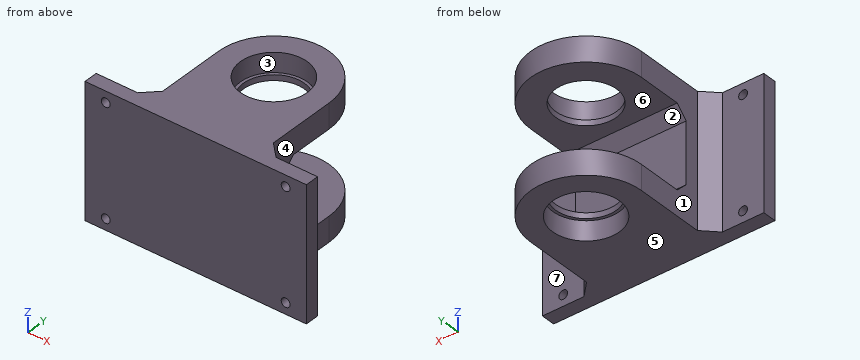
```python
from build123d import *

# Parameters (mm, degrees)
SKETCH_1_R               = 11
EXTRUDE_1_DEPTH          = 24
CUT_EXTRUDE_1_DEPTH      = 47.914816423
CUT_EXTRUDE_1_DEPTH_BACK = 47.914816423
SKETCH_2_W               = 30
SKETCH_2_H               = 69.949963181
SKETCH_4_R               = 12.05
CUT_EXTRUDE_3_DEPTH      = 7
CHAMFER_2_SIZE           = 4
SKETCH_5_W               = 48
SKETCH_5_H               = 5
EXTRUDE_2_DEPTH          = 20
CHAMFER_3_SIZE           = 5
SKETCH_6_R               = 1.6
CUT_EXTRUDE_4_DEPTH      = 73.117958928


with BuildPart() as part:
    # 草图1 → 凸台-拉伸1 (new, symmetric)
    with BuildSketch(Plane.XY):
        with BuildLine():
            Line((-20, -35), (-20, 0))
            ThreePointArc((-20, 0), (0, 20), (20, 0))
            Line((20, 0), (20, -35))
            Line((20, -35), (-20, -35))
        make_face()
        Circle(SKETCH_1_R, mode=Mode.SUBTRACT)
    extrude(amount=EXTRUDE_1_DEPTH, both=True)

    # 草图2 → 切除-拉伸1 (cut, two sides: drawn at the far end of the back side and taken through both)
    with BuildSketch(Plane(origin=(0, 0, 0), x_dir=(0, 0, -1), z_dir=(1, 0, 0)).offset(-CUT_EXTRUDE_1_DEPTH_BACK)):
        with Locations((0, 14.974981591)):
            Rectangle(SKETCH_2_W, SKETCH_2_H)
    extrude(amount=CUT_EXTRUDE_1_DEPTH + CUT_EXTRUDE_1_DEPTH_BACK, mode=Mode.SUBTRACT)

    # 草图4 → 切除-拉伸3 (cut)
    with BuildSketch(Plane(origin=(0, 0, -24), x_dir=(-1, 0, 0), z_dir=(0, 0, -1))):
        Circle(SKETCH_4_R)
    cut_extrude_3 = extrude(amount=-CUT_EXTRUDE_3_DEPTH, mode=Mode.SUBTRACT)

    # 倒角2
    chamfer_2_edges = [part.edges().sort_by_distance(p)[0] for p in [
        (0, -20, 15),
        (0, -20, -15),
    ]]
    chamfer(chamfer_2_edges, length=CHAMFER_2_SIZE)

    # 镜向1: 切除-拉伸3 across plane
    add(cut_extrude_3.mirror(Plane.XY), mode=Mode.SUBTRACT)

    # 草图5 → 凸台-拉伸2 (add)
    with BuildSketch(Plane.ZY.offset(20)):
        with Locations((0, -32.5)):
            Rectangle(SKETCH_5_W, SKETCH_5_H)
    extrude_2 = extrude(amount=EXTRUDE_2_DEPTH)

    # 镜向2: 凸台-拉伸2 across plane
    add(extrude_2.mirror(Plane.ZY))

    # 倒角3
    chamfer_3_edges = [part.edges().sort_by_distance(p)[0] for p in [
        (-20, -30, 0),
        (20, -30, 0),
    ]]
    chamfer(chamfer_3_edges, length=CHAMFER_3_SIZE)

    # 草图6 → 切除-拉伸4 (cut, through all)
    with BuildSketch(Plane.XZ.offset(35)):
        with Locations(Location((32.5, -20, 0), (0, 0, 270))):
            Circle(SKETCH_6_R)
        with Locations(Location((-32.5, -20, 0), (0, 0, 270))):
            Circle(SKETCH_6_R)
        with Locations(Location((-32.5, 20, 0), (0, 0, 270))):
            Circle(SKETCH_6_R)
        with Locations(Location((32.5, 20, 0), (0, 0, 90))):
            Circle(SKETCH_6_R)
    extrude(amount=-CUT_EXTRUDE_4_DEPTH, mode=Mode.SUBTRACT)


solid = part.part
```
Can you work these out from the model? Positions are in its coordinate system, mm. Face numbers are marked on the shaded views. A direction names the side the tool comes from. Coordinates: 2 decimals unless noted, no trailing zeros. Write each loop counter-clockwise with the first axis right and the second up, starting at its lowest first coordinate (ties: lowest second). Pieces come first, ordered by that corner, then holes. Notation, with made-up numbers: M -3,-9.75 L 14,-9.75 A8 ccw 14,5.25 Z; hole C 37.5,-23.5 d9. An arc over 180 degrees is marked long. Answer as CSV lines item,"result".
Item 1: Please list where these lines run through material, in increasing order: line 1 along X through (y, z) = (-33.2, 20); line 2 along Y through (x, z) = (0, -19); line 3 along Z through (x, y) = (-6.5, 17.5).
Geometry results:
line 1,"x = -40 to -34.1, -30.9 to 30.9, 34.1 to 40"
line 2,"y = -35 to -12.05, 12.05 to 20"
line 3,"z = -24 to -15, 15 to 24"
Item 2: Imagine slicing it at C-C on y = 7. List the corners of the cut face in (x, z) for me (3 decimals), plus the area to 3 significant figures.
Geometry results:
outline,"M -18.735,-24 L -9.808,-24 L -9.808,-17 L -8.485,-17 L -8.485,-15 L -18.735,-15 Z; M -18.735,15 L -8.485,15 L -8.485,17 L -9.808,17 L -9.808,24 L -18.735,24 Z; M 8.485,-17 L 9.808,-17 L 9.808,-24 L 18.735,-24 L 18.735,-15 L 8.485,-15 Z; M 8.485,15 L 18.735,15 L 18.735,24 L 9.808,24 L 9.808,17 L 8.485,17 Z"
area,"332 mm2"
Item 3: Imagine slicing it at B-B on z = 20. List the corners of the cut face in (x, y) for me, plus the area to 3 significant figures.
Geometry results:
outline,"M -40,-35 L -34.1,-35 L -34.1,-30 L -40,-30 Z; M -30.9,-35 L 30.9,-35 L 30.9,-30 L 25,-30 L 20,-25 L 20,0 A20 ccw -20,0 L -20,-25 L -25,-30 L -30.9,-30 Z; M 34.1,-35 L 40,-35 L 40,-30 L 34.1,-30 Z; hole C 0,0 d24.1"
area,"1,770 mm2"
Item 4: On a 3-axis mill with a long thin cutter (end or side, diameter ignored), from which of +Z, -Z, +X, -X, +Y, -Y can I reach the whole of each face in a straight line? I mean the marked faces 1, 2, 3 and 4. Say none if no direction works.
Geometry results:
face 1,"+Z, -Z, -X, +Y"
face 2,"+X, -X, +Y"
face 3,"+Z"
face 4,"+Z, -Z, +X, +Y"
Item 5: We'd pull the mould along Z, two halves only. Please class the marked faces 5, 6 and 7: +Z half, -Z half, draft (parallel to the pull), parting line (faces both ways), or undercut.
Geometry results:
face 5,"-Z half"
face 6,"undercut"
face 7,"draft"
Item 6: Imagine slicing it at D-D on z = 9. List the corners of the cut face in (x, y) for me.
Geometry results:
outline,"M -40,-35 L 40,-35 L 40,-30 L 25,-30 L 20,-25 L 20,-20 L -20,-20 L -20,-25 L -25,-30 L -40,-30 Z"
Item 7: Imagine slicing it at A-A on x = 0. List the corners of the cut face in (y, z) for me.
Geometry results:
outline,"M -35,-24 L -12.05,-24 L -12.05,-17 L -11,-17 L -11,-15 L -16,-15 L -20,-11 L -20,11 L -16,15 L -11,15 L -11,17 L -12.05,17 L -12.05,24 L -35,24 Z; M 11,-17 L 12.05,-17 L 12.05,-24 L 20,-24 L 20,-15 L 11,-15 Z; M 11,15 L 20,15 L 20,24 L 12.05,24 L 12.05,17 L 11,17 Z"
Item 8: I'm going to push flat-ended pins straight in: P1, Ø12.5, axis at y = -11, z = -4, coming from the +X side; P2, Ø4, axis at x = -32.5, z = 20, coming from the -Y side; P3, Ø7.5, axis at x = -34.5, z = 3.5, coming from the +Y side; P4, Ø2, axis at x = -20, z = -7, coming from the +Y side. Where does each tip first touch, or does it pass through?
Geometry results:
P1,"passes through"
P2,"stops at y = -35"
P3,"stops at y = -30"
P4,"stops at y = -20"
